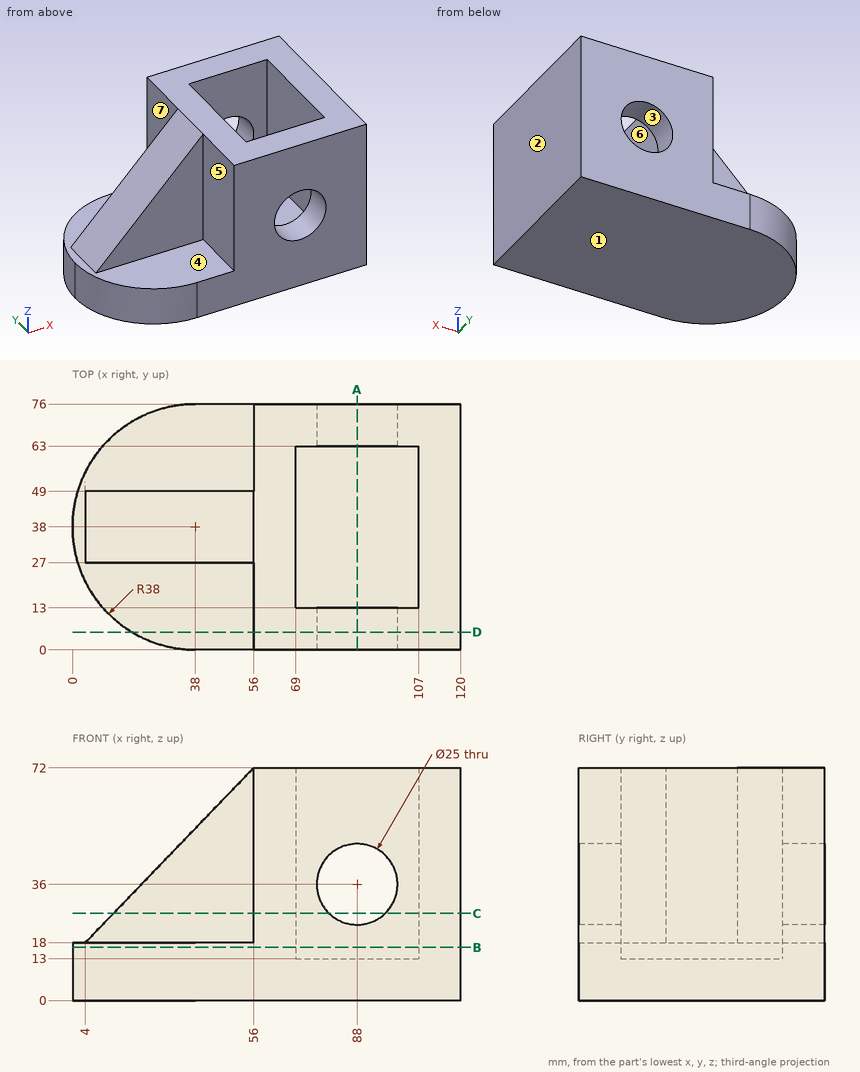
Design review of the part shown in the three views and the two pictorial views. Dimensions are in mm from the part's minimum x, y and z. A direction names the side the tool comes from. Round coordinates to 2 decimals unless told otherwise and drop trailing zeros. Write each loop counter-clockwise with the first axis right and the second up, starting at its lowest first coordinate (ties: lowest second). Pieces come first, ordered by that corner, then holes. Notation, with made-up numbers: M 51.25,56 L 91.25,56 A20 ccw 91.25,92 Z; hole C 9.5,24.5 d9. An arc over 180 degrees is marked long. Use a Markdown table: item, result. Add a question column.
Q1. We need section A-A, the plane x = 88. State the section outline as (y, z) points, plus the area to 3 significant figures.
Q2. The part is to be moulded in two halves that separate along Z. For the marked faces 1, 2 and 3, say which applies: pulls with the +Z half, pulls with the -Z half, needs draft (parallel to the pull), parting line crosses it, or undercut.
Q3. We need section C-C, the plane z = 27. State the section outline as (x, y) points, plus the area to 3 significant figures.
Q4. We need section D-D, the plane y = 5.5. State the section outline as (x, z) points, plus the area to 3 significant figures.
Q5. Machinability: for the marked faces 4, 5, 6 and 7, which of the approach directions +Z, -Z, +X, -X, +Y, -Y give a long, thin tool a straight path to every point of the face, cutting with its end or side? Answer none if there is none.
Q6. To check wall thickness, follow line 1 (Z direction, x = 88, y = 8.5); line 2 (Y direction, x = 74.5, z = 68); line 3 (X direction, y = 58.5, z = 47.5). State the ranges of each line that lie inside material, in increasing order.
Q7. We need section B-B, the plane z = 16.5. State the section outline as (x, y) points.
Q8. Insertion check: pin 1 (13.5 mm diameter, centred on y = 57.5, z = 56.5, fed in from -X); pin 2 (12 mm diameter, centred on x = 48, y = 20, fed in from +Z); pin 3 (15.5 mm diameter, centred on x = 37.5, z = 58, fed in from -Y). Each pin has a flat end and moves straight along its axis. Give the tip position at first contact, or say it passes through.
Findings below:
| question | item | result |
|---|---|---|
| 1 | outline | M 0,0 L 76,0 L 76,23.5 L 63,23.5 L 63,13 L 13,13 L 13,23.5 L 0,23.5 Z; M 0,48.5 L 13,48.5 L 13,72 L 0,72 Z; M 63,48.5 L 76,48.5 L 76,72 L 63,72 Z |
| 1 | area | 1,870 mm² |
| 2 | face 1 | pulls with the -Z half |
| 2 | face 2 | needs draft |
| 2 | face 3 | undercut |
| 3 | outline | M 12.67,27 L 56,27 L 56,0 L 79.33,0 L 79.33,13 L 69,13 L 69,63 L 79.33,63 L 79.33,76 L 56,76 L 56,49 L 12.67,49 Z; M 96.67,0 L 120,0 L 120,76 L 96.67,76 L 96.67,63 L 107,63 L 107,13 L 96.67,13 Z |
| 3 | area | 3,470 mm² |
| 4 | outline | M 18.31,0 L 120,0 L 120,72 L 56,72 L 56,18 L 18.31,18 Z; hole C 88,36 d25 |
| 4 | area | 4,800 mm² |
| 5 | face 4 | +Z, -X |
| 5 | face 5 | +Z, -X, -Y |
| 5 | face 6 | +Z |
| 5 | face 7 | +Z, -X, +Y |
| 6 | line 1 | z = 0 to 23.5, 48.5 to 72 |
| 6 | line 2 | y = 0 to 13, 63 to 76 |
| 6 | line 3 | x = 56 to 69, 107 to 120 |
| 7 | outline | M 0,38 A38 ccw 38,0 L 120,0 L 120,76 L 38,76 A38 ccw Z; hole M 69,13 L 107,13 L 107,63 L 69,63 Z |
| 8 | pin 1 | stops at x = 56 |
| 8 | pin 2 | stops at z = 18 |
| 8 | pin 3 | stops at y = 27 |
